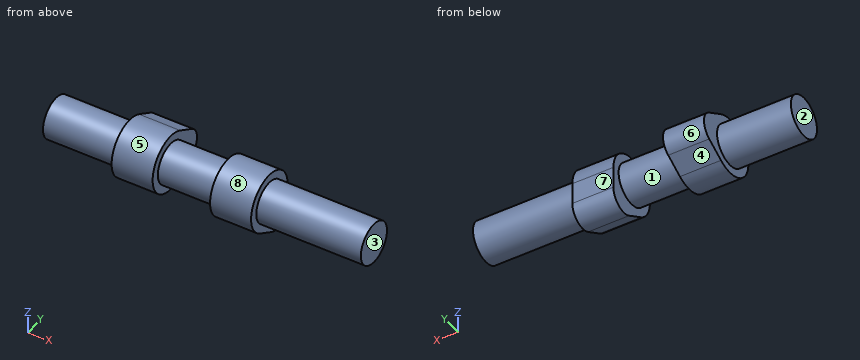
from build123d import *

# Parameters (mm, degrees)
SKETCH2_R             = 5
BOSS_EXTRUDE1_DEPTH   = 10
BODY_MOVE_COPY2_ANGLE = 60
BOSS_EXTRUDE2_START   = 28
SKETCH3_R             = 5
BOSS_EXTRUDE2_DEPTH   = 80
SKETCH4_R             = 5
CUT_EXTRUDE1_DEPTH    = 2.5


with BuildPart() as part:
    # Sketch2 → Boss-Extrude1 (new body)
    with BuildSketch(Plane.YZ):
        with BuildLine():
            Line((-3.5, -6.062177826), (1, -8.660254038))
            ThreePointArc((1, -8.660254038), (5, -8.660254038), (7, -5.196152423))
            Line((7, -5.196152423), (7, 0))
            ThreePointArc((7, 0), (-3.5, 6.062177826), (-3.5, -6.062177826))
        make_face()
        with Locations(Location((0, 0, 0), (0, 0, 270))):
            Circle(SKETCH2_R, mode=Mode.SUBTRACT)
    extrude(amount=-BOSS_EXTRUDE1_DEPTH)


with BuildPart() as body_2:
    # Body-Move/Copy1: copy of part
    add(part.part.moved(Location((-24, 0, 0))))


with BuildPart() as body_2_1:
    # Body-Move/Copy2: moved
    add(body_2.part.rotate(Axis((0, 0, 0), (1, 0, 0)), BODY_MOVE_COPY2_ANGLE))


with BuildPart() as part_1:
    add(part.part)

    add(body_2_1.part)  # Boss-Extrude2 merges body 2
    # Sketch3 → Boss-Extrude2 (add)
    with BuildSketch(Plane.YZ.offset(BOSS_EXTRUDE2_START)):
        with Locations(Location((0, 0, 0), (0, 0, 270))):
            Circle(SKETCH3_R)
    extrude(amount=-BOSS_EXTRUDE2_DEPTH)

    # Sketch4 → Cut-Extrude1 (cut)
    with BuildSketch(Plane.YZ.offset(28)):
        with Locations(Location((0, 0, 0), (0, 0, 270))):
            Circle(SKETCH4_R)
    extrude(amount=-CUT_EXTRUDE1_DEPTH, mode=Mode.SUBTRACT)


solid = part_1.part
Can you work these out from the model? Positions are in its coordinate system, mm. Face numbers are marked on the shaded views. A direction names the side the tool comes from. Give positions to 0.01 mm unless a question says otherwise; leave off trailing zeros. Loops run counter-clockwise (first coordinate to the right, second up) from the corner with the lowest first, then second, coordinate; pieces in that order, holes last. Notation, with made-up numbers: M 47.25,-18.75 L 81.25,-18.75 A32 cw 81.25,14.25 Z; hole C -27.5,13.25 d10. An arc over 180 degrees is marked long. One line per item, written item: value. Start each with the question number.
1) If we section it at B-B, the plane z = -1: Write out the boundary of the cut face in (x, y), and give its area (3 significant figures).
2) Thinking about a two-plate mould opening in X: for the marked faces 1, 2, 3 and 4, which applies, +X half, -X half, draft (parallel to the pull), parting line (faces both ways), or undercut?
3) If we section it at D-D, the plane x = 19.5: Write out the boundary of the cut face in (y, z).
4) If we section it at C-C, the plane x = -4.5: Write out the boundary of the cut face in (y, z).
5) On a 3-axis mill with a long thin cutter (end or side, diameter ignored), from which of +Z, -Z, +X, -X, +Y, -Y can I reach the whole of each face in a straight line? I mean the marked faces 5, 6, 7 and 8. Say none if no direction works.
6) If I drill on line 1 (X direction, y = 3.5, z = 4.75); line 2 (Y direction, x = -38, z = -0.25); line 3 (X direction, y = 1.75, z = -8.5), over which ranges is the centre line in solid material (lowest first)? Write a range as [from, to].
7) I'm going to push flat-ended pins straight in: pin 1 (1 mm diameter, centred on y = -1, z = 5, fed in from -X); pin 2 (1.5 mm diameter, centred on y = 7.5, z = -1.5, fed in from -X); pin 3 (1.5 mm diameter, centred on x = -5.5, z = -5.5, fed in from -Y); pin 4 (6 mm diameter, centred on x = -42, y = -2.5, fed in from +Z). Where does each tip first touch, or does it pass through?
8) If we section it at A-A, the plane y = 0: Write out the boundary of the cut face in (x, z), and give its area (3 significant figures).
Completed:
1. outline: M -52,-4.9 L -34,-4.9 L -34,-6.93 L -24,-6.93 L -24,-4.9 L -10,-4.9 L -10,-6.93 L 0,-6.93 L 0,-4.9 L 25.5,-4.9 L 25.5,4.9 L 0,4.9 L 0,7 L -10,7 L -10,4.9 L -24,4.9 L -24,9.87 L -34,9.87 L -34,4.9 L -52,4.9 Z
1. area: 871 mm^2
2. face 1: undercut
2. face 2: -X half
2. face 3: +X half
2. face 4: draft
3. outline: C 0,0 d10
4. outline: M -3.5,-6.06 L 1,-8.66 A4 ccw 7,-5.2 L 7,0 A7 ccw long Z
5. face 5: -X
5. face 6: +X, -X, +Y
5. face 7: +Z, -Z, +X, +Y
5. face 8: +X
6. line 1: x = [-34, -24], [-10, 0]
6. line 2: y = [-4.99, 4.99]
6. line 3: x = [-10, 0]
7. pin 1: stops at x = -52
7. pin 2: stops at x = -34
7. pin 3: stops at y = -5.14
7. pin 4: stops at z = 5
8. outline: M -52,-5 L -34,-5 L -34,-7 L -24,-7 L -24,-5 L -10,-5 L -10,-8.08 L 0,-8.08 L 0,-5 L 25.5,-5 L 25.5,5 L 0,5 L 0,7 L -10,7 L -10,5 L -24,5 L -24,7 L -34,7 L -34,5 L -52,5 Z
8. area: 866 mm^2
